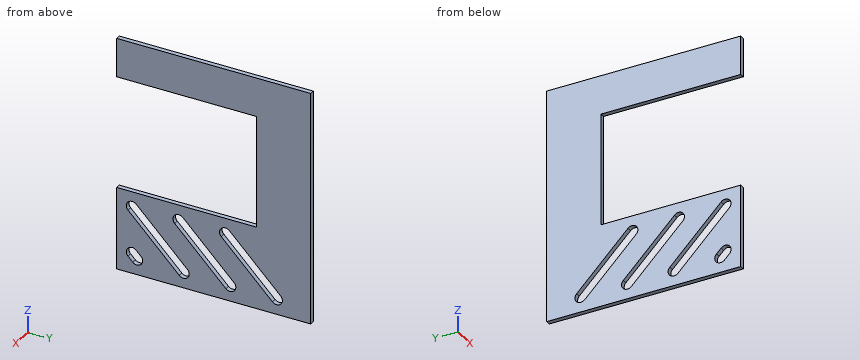
```python
from build123d import *

# Parameters (mm, degrees)
BOSS_EXTRUDE1_DEPTH = 6
SKETCH2_W           = 106
SKETCH2_H           = 107.951063415
BOSS_EXTRUDE3_DEPTH = 6
CUT_EXTRUDE1_DEPTH  = 10
LPATTERN1_COUNT     = 3
LPATTERN1_PITCH     = 60


with BuildPart() as part:
    # Sketch1 → Boss-Extrude1 (new body)
    with BuildSketch(Plane(origin=(0, 0, 0), x_dir=(0, 0, -1), z_dir=(1, 0, 0))):
        Polygon((0, 0), (50, 0), (50, 180), (194, 180), (194, 0), (300, 0), (300, 250), (0, 250), align=None)
        with BuildLine():
            Line((274.696699141, 14.696699141), (208.696699141, 80.696699141))
            ThreePointArc((208.696699141, 80.696699141), (208.696699141, 91.303300859), (219.303300859, 91.303300859))
            Line((219.303300859, 91.303300859), (285.303300859, 25.303300859))
            ThreePointArc((285.303300859, 25.303300859), (285.303300859, 14.696699141), (274.696699141, 14.696699141))
        make_face(mode=Mode.SUBTRACT)
    extrude(amount=BOSS_EXTRUDE1_DEPTH)

    # Sketch2 → Boss-Extrude3 (add)
    with BuildSketch(Plane.ZY):
        with Locations((-247, 53.975531708)):
            Rectangle(SKETCH2_W, SKETCH2_H)
    extrude(amount=-BOSS_EXTRUDE3_DEPTH)

    # Sketch3 → Cut-Extrude1 (cut)
    with BuildSketch(Plane.ZY):
        with BuildLine():
            Line((-219.303300859, 14.696699141), (-285.303300859, 80.696699141))
            ThreePointArc((-285.303300859, 80.696699141), (-285.303300859, 91.303300859), (-274.696699141, 91.303300859))
            Line((-274.696699141, 91.303300859), (-208.696699141, 25.303300859))
            ThreePointArc((-208.696699141, 25.303300859), (-208.696699141, 14.696699141), (-219.303300859, 14.696699141))
        make_face()
        with BuildLine():
            Line((-279.303300859, 14.696699141), (-285.303300859, 20.696699141))
            ThreePointArc((-285.303300859, 20.696699141), (-285.303300859, 31.303300859), (-274.696699141, 31.303300859))
            Line((-274.696699141, 31.303300859), (-268.696699141, 25.303300859))
            ThreePointArc((-268.696699141, 25.303300859), (-268.696699141, 14.696699141), (-279.303300859, 14.696699141))
        make_face()
        with BuildLine():
            Line((-214.696699141, 273.303300859), (-208.696699141, 267.303300859))
            ThreePointArc((-208.696699141, 267.303300859), (-208.696699141, 256.696699141), (-219.303300859, 256.696699141))
            Line((-219.303300859, 256.696699141), (-225.303300859, 262.696699141))
            ThreePointArc((-225.303300859, 262.696699141), (-225.303300859, 273.303300859), (-214.696699141, 273.303300859))
        make_face()
    cut_extrude1 = extrude(amount=-CUT_EXTRUDE1_DEPTH, mode=Mode.SUBTRACT)

    # LPattern1: Cut-Extrude1 ×3
    with Locations(*[(0, i * LPATTERN1_PITCH, 0) for i in range(1, LPATTERN1_COUNT)]):
        add(cut_extrude1, mode=Mode.SUBTRACT)


solid = part.part
```
Geometry check sheet. Reference: the model listing, model coordinates, mm. Coordinates: 2 decimals unless noted, no trailing zeros. Order: outer loops, then holes, each group sorted by start corner. A loop starts at its lowest first (then second) coordinate and runs counter-clockwise, first axis right, second up. Notation, with made-up numbers: M 63,6 L 67,6 A24 cw 67,30 Z; hole C 88,-29.5 d7. An arc over 180 degrees is marked long. One line per question, with ' | ' between items. Start each with the question number.
Item 1: Cross-section at C-C on x = 4. Enter the section's corners in (y, z).
Item 2: Cross-section at A-A on y = 113. Enter the section's corners in (x, z).
Item 3: Cross-section at B-B on z = -254. Enter the section's corners in (x, y).
Item 4: Material ranges on L1, parallel to Z at x = 1.5, y = 20; L2, parallel to Z at x = 0.75, y = 67; L3, parallel to Z at x = 1.5, y = 95.5, recorded low to high. Write a range as [from, to].
Item 5: Cross-section at D-D on z = -164.5. Enter the section's corners in (x, y).
Findings:
1) outline: M 0,-300 L 250,-300 L 250,0 L 0,0 L 0,-50 L 180,-50 L 180,-194 L 0,-194 Z; hole M 14.7,-279.3 L 20.7,-285.3 A7.5 ccw 31.3,-274.7 L 25.3,-268.7 A7.5 ccw Z; hole M 14.7,-219.3 L 80.7,-285.3 A7.5 ccw 91.3,-274.7 L 25.3,-208.7 A7.5 ccw Z; hole M 74.7,-219.3 L 140.7,-285.3 A7.5 ccw 151.3,-274.7 L 85.3,-208.7 A7.5 ccw Z; hole M 134.7,-219.3 L 200.7,-285.3 A7.5 ccw 211.3,-274.7 L 145.3,-208.7 A7.5 ccw Z
2) outline: M 0,-300 L 6,-300 L 6,-257.61 L 0,-257.61 Z; M 0,-236.39 L 6,-236.39 L 6,-194 L 0,-194 Z; M 0,-50 L 6,-50 L 6,0 L 0,0 Z
3) outline: M 0,0 L 6,0 L 6,49.39 L 0,49.39 Z; M 0,70.61 L 6,70.61 L 6,109.39 L 0,109.39 Z; M 0,130.61 L 6,130.61 L 6,169.39 L 0,169.39 Z; M 0,190.61 L 6,190.61 L 6,250 L 0,250 Z
4) L1: z = [-300, -284.61], [-266.5, -224.61], [-206.5, -194], [-50, 0] | L2: z = [-300, -271.61], [-250.39, -194], [-50, 0] | L3: z = [-300, -240.11], [-218.89, -194], [-50, 0]
5) outline: M 0,180 L 6,180 L 6,250 L 0,250 Z
